The listing builds one solid part. Answer for the finished solid, in the listing's coordinates (mm). Face numbers are marked on the shaded views. Round coordinates to 2 decimals unless told otherwise and drop trailing zeros. Loops run counter-clockwise (first coordinate to the right, second up) from the corner with the lowest first, then second, coordinate; pieces in that order, holes last. Notation, with made-up numbers: (68, 56) -> (104, 56) arc R22 cw to (104, 91) -> close; hole circle Ø3 at (-20.5, 78.25). An arc over 180 degrees is marked (long way). Write each question's results on one line, items separated by ' | '. Start each with the question number.
from build123d import *

# Parameters (mm, degrees)
F2_SIZE2        = 2
F2_SIZE         = 2
F3_R            = 7
F4_DEPTH        = 25
F4_COPIES_COUNT = 6


# Not quite as in the source:
# - a pattern or mirror of a feature is missing from the dataset's text; its kind, count and spacing are read off the source's solid


with BuildPart() as f1:
    # F0 (on Right) → F1 (revolve)
    with BuildSketch(Plane.YZ):
        with BuildLine():
            Line((92, 16), (0, 16))
            Line((0, 16), (0, 8))
            Line((0, 8), (43, 8))
            ThreePointArc((43, 8), (44.4142135624, 7.4142135624), (45, 6))
            Line((45, 6), (45, 0))
            Line((45, 0), (80, 0))
            Line((80, 0), (89.0352761804, 2.4209949559))
            ThreePointArc((89.0352761804, 2.4209949559), (91.1734133612, 3.8496525451), (92, 6.2846982611))
            Line((92, 6.2846982611), (92, 16))
        make_face()
    revolve(axis=Axis((0, 0, 0.8759116049), (0, 0, -1)))

    # F2
    f2_edges = [f1.edges().sort_by_distance(p)[0] for p in [
        (0, -45, 0),
    ]]
    chamfer(f2_edges, length=F2_SIZE, length2=F2_SIZE2)

    # F3 (on face) → F4 (cut)
    with BuildSketch(Plane(origin=(0, 0, 0), x_dir=(1, 0, 0), z_dir=(0, 0, -1))):
        with Locations((0, 65)):
            Circle(F3_R)
    f4 = extrude(amount=-F4_DEPTH, mode=Mode.SUBTRACT)

    # F4_copies: F4 ×6 about axis
    f4_copies_axis = Axis((0, 0, 0), (0, 0, 1))
    for i in range(1, F4_COPIES_COUNT):
        add(f4.rotate(f4_copies_axis, i * 360 / F4_COPIES_COUNT), mode=Mode.SUBTRACT)


solid = f1.part
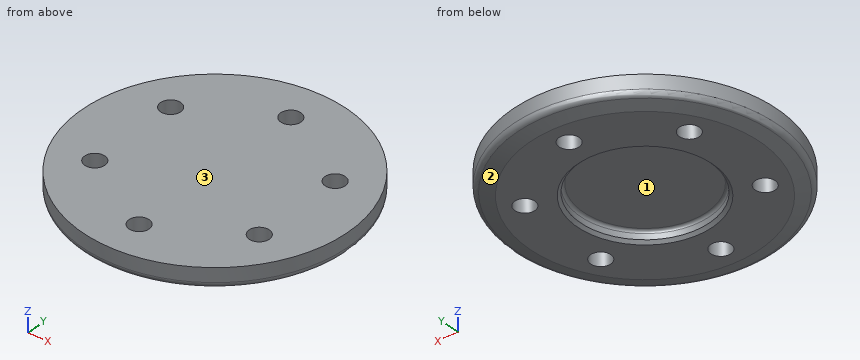
Item 1: The part is cut by section A-A, the plane x = 0. Give the vertices of the cut face in (y, z), plus the area to 3 significant figures.
Item 2: The part is cut by section B-B, the plane z = 10.25. Give the vertices of the cut face in (x, y).
Item 3: Each of these flat-tipped pins is pushed along its axis until it touches: pin 1 Ø1 at (x, z) = (-69, 3.5) entering from +Y; pin 2 Ø5 at (x, z) = (6.5, 7.5) entering from -Y; pin 3 Ø6 at (y, z) = (33, 11) entering from -X. Where does it stop, or does it pass through?
Item 4: The part is cut by section C-C, the plane y = -32.5. Give the number of separate pieces and of enclosed holes in the cut face, plus the area to 3 significant figures.
Item 5: Straight lines are drawn through the part: L1, parallel to X at y = -32.5, z = 3.75; L2, parallel to Y at x = -58, z = 9.5; L3, parallel to Z at x = 12, y = 20. For each, find the intervals that lie inside material, in ascending order. Write a range as [from, to].
Item 6: Determine the mould class of the marked faces 1, 2 and 3 for opening direction Y: +Y half, -Y half, draft (parallel to the pull), parting line (faces both ways), or undercut.
Report:
1) outline: (-92, 6.28) arc R4 ccw to (-89.04, 2.42) -> (-80, 0) -> (-72, 0) -> (-72, 16) -> (-92, 16) -> close; (-58, 0) -> (-47, 0) -> (-45, 2) -> (-45, 6) arc R2 cw to (-43, 8) -> (43, 8) arc R2 cw to (45, 6) -> (45, 2) -> (47, 0) -> (58, 0) -> (58, 16) -> (-58, 16) -> close; (72, 0) -> (80, 0) -> (89.04, 2.42) arc R4 ccw to (92, 6.28) -> (92, 16) -> (72, 16) -> close | area: 1,730 mm2
2) outline: circle Ø184 at (0, 0); hole circle Ø14 at (-56.29, -32.5); hole circle Ø14 at (-56.29, 32.5); hole circle Ø14 at (0, -65); hole circle Ø14 at (0, 65); hole circle Ø14 at (56.29, -32.5); hole circle Ø14 at (56.29, 32.5)
3) pin 1: stops at y = 60.01 | pin 2: stops at y = -91.91 | pin 3: stops at x = -86.97
4) separate pieces: 3 | enclosed holes: 0 | area: 1,760 mm2
5) L1: x = [-85.1, -63.29], [-49.29, -31.12], [31.12, 49.29], [63.29, 85.1] | L2: y = [-71.41, -39.29], [-25.71, 25.71], [39.29, 71.41] | L3: z = [8, 16]
6) face 1: undercut | face 2: parting line | face 3: draft
